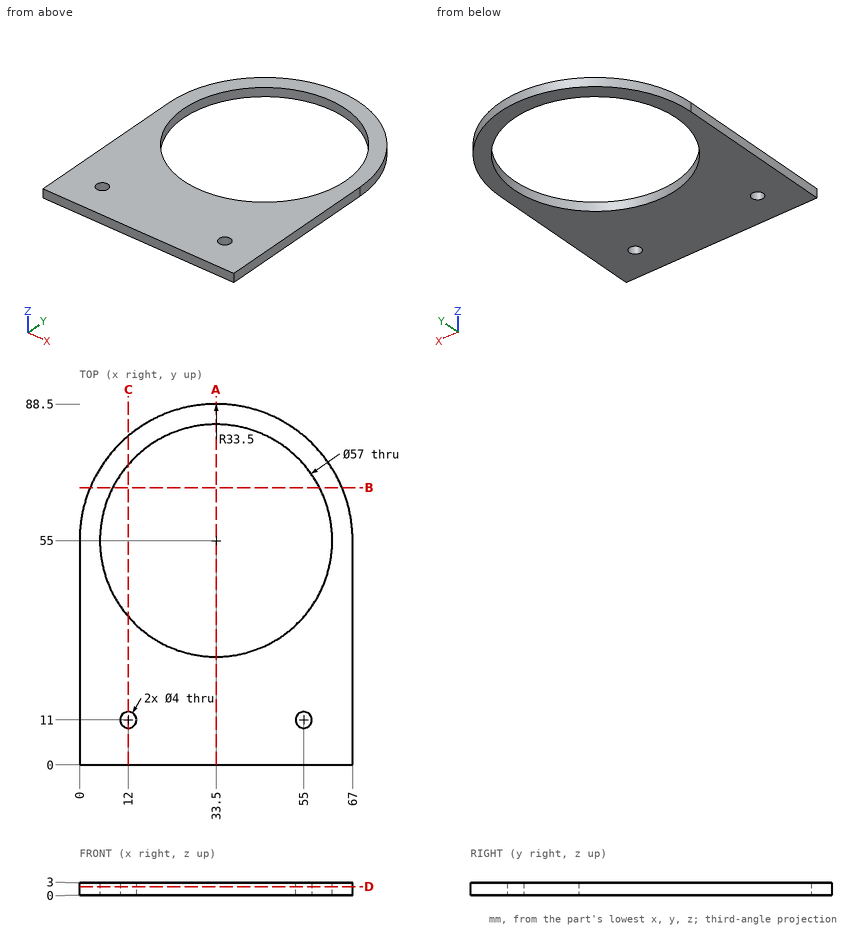
Job drawing, mm, ordinate dimensions from the low corner. One solid piece. Round coordinates to 2 decimals unless told otherwise and drop trailing zeros. Order: outer loops, then holes, each group sorted by start corner. A loop starts at its lowest first (then second) coordinate and runs counter-clockwise, first axis right, second up. Notation, with made-up numbers: (88.25, 10) - (145.25, 10) arc R24 cw to (145.25, 20) - close; hole circle Ø6 at (15.5, -11). An arc over 180 degrees is marked (long way). Use CSV: the item, a comma, the result in double quotes. Start each with the question number.
1) Wall check: L1, parallel to Y at x = 33.5, z = 0.75; L2, parallel to Y at x = 12, z = 1.65; L3, parallel to X at y = 56, z = 1.45. Give the ranges that are in metal, low to high. Write a range as [from, to].
2) Saw through at A-A (x = 33.5). List the corners of the cut face in (y, z).
3) Saw through at C-C (x = 12). List the corners of the cut face in (y, z).
4) Saw through at D-D (z = 2.05). List the corners of the cut face in (x, y).
5) Saw through at B-B (y = 68). List the corners of the cut face in (x, z).
6) Pin check, flat tip, straight feed: pin 1 Ø3 at (x, y) = (55, 11) entering from +Z. Stop position of the tip, or through.
Values follow:
1,L1,"y = [0, 26.5], [83.5, 88.5]"
1,L2,"y = [0, 9], [13, 36.29], [73.71, 80.69]"
1,L3,"x = [0.01, 5.02], [61.98, 66.99]"
2,outline,"(0, 0) - (26.5, 0) - (26.5, 3) - (0, 3) - close; (83.5, 0) - (88.5, 0) - (88.5, 3) - (83.5, 3) - close"
3,outline,"(0, 0) - (9, 0) - (9, 3) - (0, 3) - close; (13, 0) - (36.29, 0) - (36.29, 3) - (13, 3) - close; (73.71, 0) - (80.69, 0) - (80.69, 3) - (73.71, 3) - close"
4,outline,"(0, 0) - (67, 0) - (67, 55) arc R33.5 ccw to (0, 55) - close; hole circle Ø57 at (33.5, 55); hole circle Ø4 at (12, 11); hole circle Ø4 at (55, 11)"
5,outline,"(2.63, 0) - (8.14, 0) - (8.14, 3) - (2.63, 3) - close; (58.86, 0) - (64.37, 0) - (64.37, 3) - (58.86, 3) - close"
6,pin 1,"passes through"
